Read the model definition and answer for the solid it produces. Units are mm, in the model's axes. Face numbers are marked on the shaded views. Give positions to 0.01 mm unless a question says otherwise; leave off trailing zeros. Loops run counter-clockwise (first coordinate to the right, second up) from the corner with the lowest first, then second, coordinate; pieces in that order, holes last. Notation, with made-up numbers: (50.25, 52) -> (62.25, 52) arc R8 ccw to (62.25, 63) -> close; hole circle Ø8 at (17.5, -12.75). An arc over 180 degrees is marked (long way). Write each question's results on one line, items separated by ' | '. Start each with the question number.
Item 1: Section C-C on x = -17.5 is taken. Write down the section's boundary in (y, z).
Item 2: Determine the mould class of the marked faces 1, 2, 3 and 4 for opening direction Z: +Z half, -Z half, draft (parallel to the pull), parting line (faces both ways), or undercut.
Item 3: Section A-A on y = 2.05 is taken. Write down the section's boundary in (x, z), and give its area (3 significant figures).
Item 4: Section B-B on z = 0 is taken. Write down the section's boundary in (x, y).
Item 5: Find the intervals of material crossed by line 1 (X direction, y = 0.65, z = 8.75); line 2 (X direction, y = 0.7, z = 0); line 3 (Z direction, x = 3, y = 2.75), in increasing order.
Item 6: Each of these flat-tipped pins is pushed along its axis until it touches: P1, Ø10, axis at x = -18, z = 9.5, coming from the -Y side; P2, Ø2, axis at x = 1.68, z = -8.75, coming from the +Y side. Where does it stop, or does it pass through?
```python
from build123d import *

# Parameters (mm, degrees)
SKETCH1_W           = 32.429536638
SKETCH1_H           = 25.007766804
SKETCH1_R           = 1.75
SKETCH1_R_2         = 5.5
BOSS_EXTRUDE1_DEPTH = 3


with BuildPart() as part:
    # Sketch1 → Boss-Extrude1 (new body)
    with BuildSketch(Plane(origin=(0, 0, 0), x_dir=(1, 0, 0), z_dir=(0, 1, 0))):
        with Locations((-9.865681564, 0)):
            Rectangle(SKETCH1_W, SKETCH1_H)
        with Locations((1.678034292, -8.75)):
            Circle(SKETCH1_R, mode=Mode.SUBTRACT)
        with Locations((1.678034292, 8.75)):
            Circle(SKETCH1_R, mode=Mode.SUBTRACT)
        with Locations((-18.921965708, 0)):
            Circle(SKETCH1_R_2, mode=Mode.SUBTRACT)
    extrude(amount=BOSS_EXTRUDE1_DEPTH)


solid = part.part
```
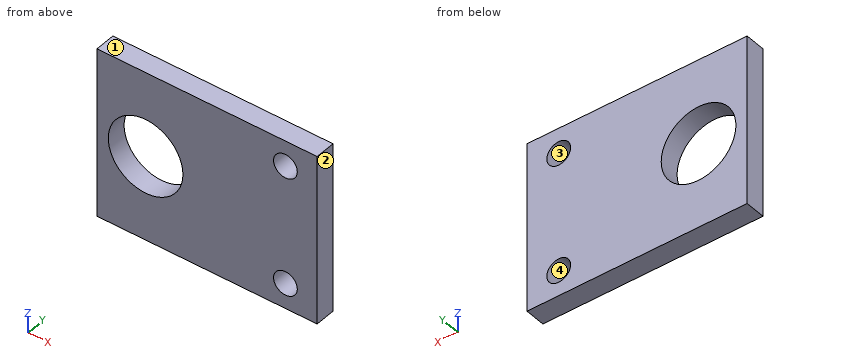
Findings:
1) outline: (0, -12.5) -> (3, -12.5) -> (3, -5.31) -> (0, -5.31) -> close; (0, 5.31) -> (3, 5.31) -> (3, 12.5) -> (0, 12.5) -> close
2) face 1: +Z half | face 2: draft | face 3: undercut | face 4: undercut
3) outline: (-26.08, -12.5) -> (6.35, -12.5) -> (6.35, 12.5) -> (-26.08, 12.5) -> close; hole circle Ø11 at (-18.92, 0); hole circle Ø3.5 at (1.68, -8.75); hole circle Ø3.5 at (1.68, 8.75) | area: 697 mm2
4) outline: (-26.08, 0) -> (-24.42, 0) -> (-24.42, 3) -> (-26.08, 3) -> close; (-13.42, 0) -> (6.35, 0) -> (6.35, 3) -> (-13.42, 3) -> close
5) line 1: -26.08 to -0.07, 3.43 to 6.35 | line 2: -26.08 to -24.42, -13.42 to 6.35 | line 3: -12.5 to -9.9, -7.6 to 7.6, 9.9 to 12.5
6) P1: y = 0 | P2: through
